from build123d import *

# Parameters (mm, degrees)
F0_W           = 480
F0_H           = 150
F1_DEPTH       = 20
F2_D           = 10.5
F2_DEPTH       = 35
F2_CBORE_D     = 25
F2_CBORE_DEPTH = 12
F2_TIP         = 3.1545182499
F3_D           = 8
F3_DEPTH       = 35
F3_TIP         = 2.4034424761


with BuildPart() as f1:
    # F0 (on Front) → F1 (new body)
    with BuildSketch(Plane.XZ):
        with Locations((240, 75)):
            Rectangle(F0_W, F0_H)
    extrude(amount=F1_DEPTH)

    # F2
    with Locations(Plane(origin=(0, 0, 0), x_dir=(1, 0, 0), z_dir=(0, 1, 0))):
        with Locations((435, -126), (435, -24), (45, -126), (45, -24)):
            CounterBoreHole(F2_D / 2, F2_CBORE_D / 2, F2_CBORE_DEPTH, depth=F2_DEPTH)
            with Locations((0, 0, -(F2_DEPTH + F2_TIP / 2))):  # 118° drill point
                Cone(0, F2_D / 2, F2_TIP, mode=Mode.SUBTRACT)

    # F3
    with Locations(Plane(origin=(0, 0, 0), x_dir=(1, 0, 0), z_dir=(0, 1, 0))):
        with Locations((115, -125), (115, -25), (365, -25), (365, -125)):
            Hole(F3_D / 2, depth=F3_DEPTH)
            with Locations((0, 0, -(F3_DEPTH + F3_TIP / 2))):  # 118° drill point
                Cone(0, F3_D / 2, F3_TIP, mode=Mode.SUBTRACT)


solid = f1.part
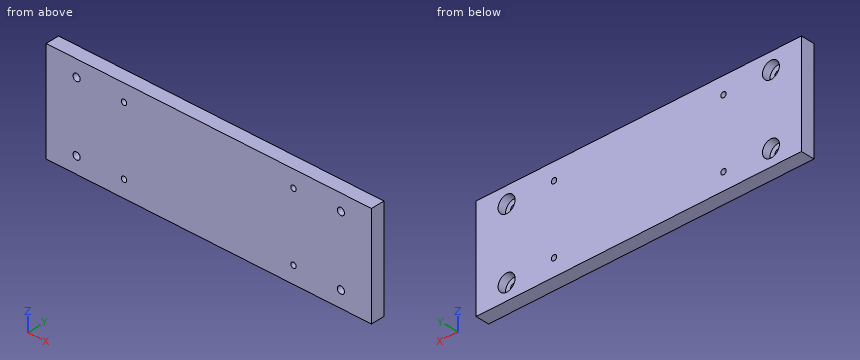
Design review of the part built by this model. Coordinates are the model's own, in mm. Round coordinates to 2 decimals unless told otherwise and drop trailing zeros. Loops run counter-clockwise (first coordinate to the right, second up) from the corner with the lowest first, then second, coordinate; pieces in that order, holes last. Notation, with made-up numbers: M 51,52.25 L 78,52.25 A20 ccw 78,63.25 Z; hole C 15.25,67 d7. An arc over 180 degrees is marked long. Answer as a JSON object with one key per item and string values.
Item 1: Wall thickness on L1, parallel to Z at x = 45.5, y = -19; L2, parallel to X at y = -13.75, z = 25; L3, parallel to Z at x = 45, y = -3.75: over which ranges is each line inside the solid? List them lowest first. Write a range as from..to.
Answer sheet:
{"L1": "z = 0..18.77, 29.23..120.77, 131.23..150", "L2": "x = 0..39.85, 50.15..111, 119..361, 369..429.85, 440.15..480", "L3": "z = 0..11.5, 36.5..113.5, 138.5..150"}
Item 2: Clearance check with flat-ended pins moving along their axes: P1, Ø20, axis at x = 435.5, z = 25.5, coming from the +Y side; P2, Ø6.5, axis at x = 365, z = 125, coming from the -Y side. State where each tip first meets the part, or that it passes through.
Answer sheet:
{"P1": "stops at y = -12", "P2": "passes through"}
Item 3: We need section B-B on x = 435. Give the boundary of the cut face in (y, z).
Answer sheet:
{"outline": "M -20,0 L 0,0 L 0,11.5 L -12,11.5 L -12,18.75 L -20,18.75 Z; M -20,29.25 L -12,29.25 L -12,36.5 L 0,36.5 L 0,113.5 L -12,113.5 L -12,120.75 L -20,120.75 Z; M -20,131.25 L -12,131.25 L -12,138.5 L 0,138.5 L 0,150 L -20,150 Z"}
Item 4: We need section A-A on y = -5. State how many separate pieces and enclosed holes the cut face has, and give its area (3 significant figures).
Answer sheet:
{"separate pieces": "1", "enclosed holes": "8", "area": "69,800 mm^2"}
